Autodesk Inventor part; units mm, degrees
ref_plane "it_schrschei_st_XY" through (7.5, 0, 0) normal (1, 0, 0) x (0, 0, -1)
ref_plane "it_schrschei_st_YZ" through (7.5, 0, 0) normal (0, 0, -1) x (0, 1, 0)
ref_plane "it_schrschei_st_ZX" through (7.5, 0, 0) normal (0, 1, 0) x (1, 0, 0)
sketch "Sketch_5" plane through (0, 0, 0) normal (0, 0, 1) x (1, 0, 0)
  line L0 (500, 0) -> (-500, 0)
  line L1 (2.5, 8.4) -> (2.5, 7)
  line L2 (2.5, 7) -> (12.5, 7)
  line L3 (12.5, 7) -> (12.5, 8.4)
  line L4 (12.5, 8.4) -> (7.5, 10)
  line L5 (7.5, 10) -> (2.5, 8.4)
revolve "Revolution1" add sketch "Sketch_5" angle 360 about axis through (500, 0, 0) along (1, 0, 0)
sketch "Sketch_6" plane through (7.5, 0, 0) normal (1, 0, 0) x (0, 0, -1)
  line L0 (-0.85, -10) -> (0.85, -10)
  line L1 (0.85, -10) -> (0.85, -6.5)
  line L2 (0.85, -6.5) -> (-0.85, -6.5)
  line L3 (-0.85, -6.5) -> (-0.85, -10)
extrude "Extrusion1" cut sketch "Sketch_6" along normal mid plane 15
ref_plane "it_schrschei_st_XY" through (7.5, 0, 0) normal (1, 0, 0) x (0, 0, -1)
ref_plane "it_schrschei_st_YZ" through (7.5, 0, 0) normal (0, 0, -1) x (0, 1, 0)
ref_plane "it_schrschei_st_ZX" through (7.5, 0, 0) normal (0, 1, 0) x (1, 0, 0)
properties part number "61581400_3"
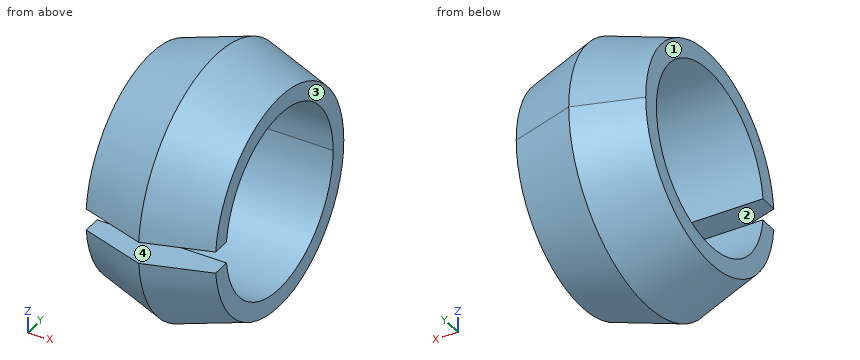
Geometry: final body of the model. Coordinates: model frame, mm. Face numbers are marked on the shaded views. A direction names the side the tool comes from. Coordinates: 2 decimals unless noted, no trailing zeros. Write each loop counter-clockwise with the first axis right and the second up, starting at its lowest first coordinate (ties: lowest second). Pieces come first, ordered by that corner, then holes. Notation, with made-up numbers: M 3.25,-26.75 L 28.25,-26.75 A22 ccw 28.25,3.25 Z; hole C -17,82 d4. An arc over 180 degrees is marked long. Use CSV: the item, a comma, the result in double quotes. Start each with the question number.
1. First-contact query: P1, Ø6, axis at x = 5, z = -5.5, coming from the -Y side; P2, Ø4, axis at x = 3.5, y = 6.5, coming from the +Z side; P3, Ø0.9, axis at x = 5.5, y = -8, coming from the +Z side. Flat tips, straight axial feed; report the tip coordinate or a pass-through.
2. Cut plane C-C on x = 11.25. Return the cut outline in (y, z).
3. Cut plane B-B on x = 5.25. Return the cut outline in (y, z).
4. Cut plane A-A on y = 0. Return the cut outline in (x, z), plus the area to 3 significant figures.
5. Mould query, pull axis Z, two halves, no side actions, for the marked faces 3 and 4. Classes: pulls with the +Z half, pulls with the -Z half, needs draft (parallel to the pull), parting line crosses it, or undercut.
6. Reachability of the marked faces 1 and 2 from +Z, -Z, +X, -X, +Y, -Y: full face, straight path, thin tool, end or side. Return the list, or none.
7. Ray query, probe 1 along Y at (x, z) = (8, -1.25); probe 2 along Z at (x, y) = (4.25, 5.25); probe 3 along Y at (x, z) = (12.25, 5.5). Return the intervals inside material, ascending.
Entries:
1,P1,"y = -9.28"
1,P2,"z = 7.68"
1,P3,"z = 5.58"
2,outline,"M -8.76,-0.85 A8.8 ccw long -8.76,0.85 L -6.95,0.85 A7 cw long -6.95,-0.85 Z"
3,outline,"M -9.24,-0.85 A9.28 ccw long -9.24,0.85 L -6.95,0.85 A7 cw long -6.95,-0.85 Z"
4,outline,"M 2.5,-8.4 L 7.5,-10 L 12.5,-8.4 L 12.5,-7 L 2.5,-7 Z; M 2.5,7 L 12.5,7 L 12.5,8.4 L 7.5,10 L 2.5,8.4 Z"
4,area,"44.0 mm²"
5,face 3,"needs draft"
5,face 4,"undercut"
6,face 1,"+Z, -Z, -X, +Y, -Y"
6,face 2,"+X, -X, -Y"
7,probe 1,"-9.76 to -6.89, 6.89 to 9.76"
7,probe 2,"-7.26 to -4.63, 4.63 to 7.26"
7,probe 3,"-6.45 to -4.33, 4.33 to 6.45"
